from build123d import *

# Parameters (mm, degrees)
BOSS_EXTRUDE1_DEPTH = 0.25
BOSS_EXTRUDE2_DEPTH = 0.25
CUT_EXTRUDE1_DEPTH  = 6.593003707
CUT_EXTRUDE2_DEPTH  = 6.593003707
DRAFT1_ANGLE        = 34.486089424
DRAFT2_ANGLE        = 50.980599525
DRAFT3_ANGLE        = 16.594713156
DRAFT4_ANGLE        = -16.43287546
DRAFT5_ANGLE        = 50.980599525
SKETCH5_W           = 0.16
SKETCH5_H           = 0.25
CHAMFER1_SIZE       = 0.063800239
FILLET1_R           = 0.2
FILLET2_R           = 0.544507155
FILLET3_R           = 0.697211686


with BuildPart() as part:
    # Sketch1 → Boss-Extrude1 (new body)
    with BuildSketch(Plane(origin=(0, 0, -0.125), x_dir=(-1, 0, 0), z_dir=(0, 0, -1))):
        with BuildLine():
            Line((-0.272408935, -3.667083787), (0.272408935, -3.667083787))
            Line((0.272408935, -3.667083787), (0.272408935, -4.143899332))
            Line((0.272408935, -4.143899332), (0.873103994, -4.143899332))
            Line((0.873103994, -4.143899332), (1.051569895, -3.965092957))
            Line((1.051569895, -3.965092957), (0.506698534, -3.965092957))
            Line((0.506698534, -3.965092957), (0.506698534, -3.283729886))
            ThreePointArc((0.506698534, -3.283729886), (0.259096573, -3.03452958), (0.179431493, -2.692387798))
            Line((0.179431493, -2.692387798), (0.290781228, -0.37153351))
            Line((0.290781228, -0.37153351), (1.835162636, 0.252738405))
            Line((1.835162636, 0.252738405), (2.536874566, -0.443310952))
            Line((2.536874566, -0.443310952), (3.165693689, 0.190623805))
            Line((3.165693689, 0.190623805), (2.398976763, 0.95115359))
            Line((2.398976763, 0.95115359), (1.838429548, 0.613387961))
            ThreePointArc((1.838429548, 0.613387961), (0.12624114, 0.405056697), (-1.168932242, 1.544142722))
            Line((-1.168932242, 1.544142722), (-1.729686411, -0.337503893))
            Line((-1.729686411, -0.337503893), (-1.821011369, -0.310568547))
            Line((-1.821011369, -0.310568547), (-1.821011369, 0.484030911))
            Line((-1.821011369, 0.484030911), (-2.056654947, 0.484030911))
            Line((-2.056654947, 0.484030911), (-2.056654947, -0.607371456))
            Line((-2.056654947, -0.607371456), (-1.482657454, -0.77842987))
            ThreePointArc((-1.482657454, -0.77842987), (-0.858095498, -0.237884247), (-0.269395252, -0.817279818))
            Line((-0.269395252, -0.817279818), (-0.179431493, -2.692387798))
            add(Edge.make_bspline(
                [(-0.179431493, -2.723199698), (-0.179183719, -2.712865075), (-0.179186918, -2.702588974), (-0.179431493, -2.692387798)],
                knots=[0, 0, 0, 0, 1, 1, 1, 1], degree=3))
            add(Edge.make_bspline(
                [(-0.507437255, -3.283729886), (-0.319927849, -3.178374639), (-0.179431493, -2.941093516), (-0.179431493, -2.723199698)],
                knots=[0, 0, 0, 0, 1, 1, 1, 1], degree=3))
            Line((-0.507437255, -3.283729886), (-0.507437255, -3.965092957))
            Line((-0.507437255, -3.965092957), (-1.051569895, -3.965092957))
            Line((-1.051569895, -3.965092957), (-0.628774335, -4.388695119))
            Line((-0.628774335, -4.388695119), (-0.272408935, -4.143899332))
            Line((-0.272408935, -4.143899332), (-0.272408935, -3.667083787))
        make_face()
    extrude(amount=-BOSS_EXTRUDE1_DEPTH)

    # Sketch2 → Boss-Extrude2 (add)
    with BuildSketch(Plane(origin=(0, 0, -0.125), x_dir=(-1, 0, 0), z_dir=(0, 0, -1))):
        Polygon((-0.129661741, -3.146789365), (0.129661741, -3.146789365), (0.129661741, -4.454012909), (0, -4.58367465), (-0.129661741, -4.454012909), align=None)
    extrude(amount=BOSS_EXTRUDE2_DEPTH)

    # Sketch3 → Cut-Extrude1 (cut, through all)
    with BuildSketch(Plane.XY.offset(0.125)):
        Polygon((-2.195377886, 0.828472215), (-2.794411885, 0.234272214), (-2.56905624, 0.007083233), (-1.912701402, 0.658141514), align=None)
    extrude(amount=-CUT_EXTRUDE1_DEPTH, mode=Mode.SUBTRACT)

    # Sketch4 → Cut-Extrude2 (cut, through all)
    with BuildSketch(Plane.XY.offset(0.125)):
        with BuildLine():
            Line((1.465134235, 0.550217916), (1.168932242, 1.544142722))
            ThreePointArc((1.168932242, 1.544142722), (0.534119283, 0.746589992), (-0.400581525, 0.339880942))
            ThreePointArc((-0.400581525, 0.339880942), (-0.007751749, 0.365487208), (0.382199804, 0.311554845))
            ThreePointArc((0.382199804, 0.311554845), (0.951331817, 0.305357276), (1.465134235, 0.550217916))
        make_face()
    extrude(amount=-CUT_EXTRUDE2_DEPTH, mode=Mode.SUBTRACT)

    # Draft1
    draft1_faces = [part.faces().sort_by_distance(p)[0] for p in [
        (-0.572756465, -4.143899332, 0),
    ]]
    draft(draft1_faces, Plane(origin=(-0.272408935, -3.667083787, 0.125), x_dir=(0, 0, 1), z_dir=(1, 0, 0)), DRAFT1_ANGLE)

    # Draft2
    draft2_faces = [part.faces().sort_by_distance(p)[0] for p in [
        (-0.779134215, -3.965092957, 0),
    ]]
    draft(draft2_faces, Plane(origin=(-0.506698534, -3.965092957, 0.125), x_dir=(0, -1, 0), z_dir=(-1, 0, 0)), DRAFT2_ANGLE)

    # Draft3
    draft3_faces = [part.faces().sort_by_distance(p)[0] for p in [
        (2.056654947, -0.061670272, 0),
    ]]
    draft(draft3_faces, Plane(origin=(1.821011369, 0.484030911, 0.125), x_dir=(1, 0, 0), z_dir=(0, 1, 0)), DRAFT3_ANGLE)

    # Draft4
    draft4_faces = [part.faces().sort_by_distance(p)[0] for p in [
        (1.821011369, 0.086731182, 0),
    ]]
    draft(draft4_faces, Plane(origin=(1.821011369, 0.484030911, 0.125), x_dir=(1, 0, 0), z_dir=(0, 1, 0)), DRAFT4_ANGLE)

    # Draft5
    draft5_faces = [part.faces().sort_by_distance(p)[0] for p in [
        (0.779503575, -3.965092957, 0),
    ]]
    draft(draft5_faces, Plane(origin=(0.507437255, -3.283729886, 0.125), x_dir=(0, 1, 0), z_dir=(1, 0, 0)), DRAFT5_ANGLE)

    # Sketch5 → Revolve1 (revolve)
    with BuildSketch(Plane.XZ.offset(3.286499627), mode=Mode.PRIVATE) as revolve1_sk:
        with Locations((0.08, 0.25)):
            Rectangle(SKETCH5_W, SKETCH5_H)
    revolve(revolve1_sk.sketch.rotate(Axis((0, -3.286499627, 0.375), (0, 0, -1)), 180), axis=Axis((0, -3.286499627, 0.375), (0, 0, -1)))

    # Sketch6 → Revolve2 (revolve)
    with BuildSketch(Plane.XZ, mode=Mode.PRIVATE) as revolve2_sk:
        Polygon((0.1, 0.875), (0, 0.875), (0, 0.125), (0.2, 0.125), (0.2, 0.375), (0.1, 0.375), align=None)
    revolve(revolve2_sk.sketch.rotate(Axis((0, 0, 0.875), (0, 0, -1)), 180), axis=Axis((0, 0, 0.875), (0, 0, -1)))

    # Sketch7 → Revolve3 (revolve)
    with BuildSketch(Plane(origin=(0, 0, 0), x_dir=(1, 0, 0), z_dir=(0, 1, 0))):
        Polygon((0.12, 1.125), (0, 1.125), (0, 0.125), (0.3, 0.125), (0.3, 0.625), (0.12, 0.625), align=None)
    revolve(axis=Axis((0, 0, -1.125), (0, 0, 1)))

    # Chamfer1
    # the kernel refuses this chamfer: 0.098147605, 0.063800239 mm, written as the material it takes off along each edge
    with BuildSketch(Plane(origin=(1.465134235, 0.550217916, 0.391937228), x_dir=(0.28559993905101894, -0.9583489316600996, 0), z_dir=(0, 0, -1))) as chamfer1_piece_1:
        with BuildLine():
            Line((CHAMFER1_SIZE * 1.00000000412, 0), (0.034717393, 0.097589357))
            ThreePointArc((0.034717393, 0.097589357), (0.018892926, 0.049933601), (0, 0))
            Line((0, 0), (CHAMFER1_SIZE * 1.00000000412, 0))
        make_face()
    extrude(amount=0.783874457, mode=Mode.SUBTRACT)

    # Fillet1
    fillet1_edges = [part.edges().sort_by_distance(p)[0] for p in [
        (1.482657454, -0.77842987, 0),
        (-2.536874566, -0.443310952, 0),
    ]]
    fillet(fillet1_edges, radius=FILLET1_R)

    # Fillet2
    fillet2_edges = [part.edges().sort_by_distance(p)[0] for p in [
        (-1.835162636, 0.252738405, 0),
    ]]
    fillet(fillet2_edges, radius=FILLET2_R)

    # Fillet3
    fillet3_edges = [part.edges().sort_by_distance(p)[0] for p in [
        (-0.290781228, -0.37153351, 0),
    ]]
    fillet(fillet3_edges, radius=FILLET3_R)


solid = part.part
Could you check a few things on this model? Use its own coordinates, in mm. Coordinates: 2 decimals unless noted, no trailing zeros. Order: outer loops, then holes, each group sorted by start corner. A loop starts at its lowest first (then second) coordinate and runs counter-clockwise, first axis right, second up.
Q1. Suppose I cut it at C-C on z = -0.5. Please give me the cut outline in (x, y).
Q2. Please list where these lines run through material, in increasing order: L1, parallel to X at y = -4.3, z = -0.3; L2, parallel to Z at x = -2.15, y = 0.05 (3 decimals); L3, parallel to X at y = -3.5, z = 0.
Q3. Will these pins go through, and if not, where does the flat tip stop? pin 1 (2 mm diameter, centred on x = -1, y = -2.5, fed in from -Z) (3 decimals); pin 2 (1 mm diameter, centred on x = 0, y = -3, fed in from -Z) (3 decimals).
Q4. Suppose I cut it at A-A on y = -3.8. Please give me the cut outline in (x, z) (3 decimals), and give its area (3 significant figures).
Q5. Suppose I cut it at B-B on z = 0.5. Please give me the cut outline in (x, y), and give its area (3 significant figures).
Answer:
1. outline: circle Ø0.6 at (0, 0)
2. L1: x = -0.13 to 0.13
2. L2: z = -0.125 to 0.125
2. L3: x = -0.51 to 0.51
3. pin 1: stops at z = -0.125
3. pin 2: stops at z = -0.375
4. outline: (-0.507, -0.125) - (-0.272, -0.125) - (-0.272, 0.125) - (-0.507, 0.125) - close; (-0.13, -0.375) - (0.13, -0.375) - (0.13, -0.125) - (-0.13, -0.125) - close; (0.272, -0.125) - (0.507, -0.125) - (0.507, 0.125) - (0.272, 0.125) - close
4. area: 0.182 mm2
5. outline: circle Ø0.2 at (0, 0)
5. area: 0.0314 mm2
